```python
from build123d import *

# Parameters (mm, degrees)
SKETCH1_W                = 13
SKETCH1_H                = 6.8
BOSS_EXTRUDE1_DEPTH      = 6.4
SKETCH2_W                = 3.286897276
SKETCH2_H                = 0.917770019
SKETCH2_W_2              = 3.564362631
BOSS_EXTRUDE2_DEPTH      = 0.1
BOSS_EXTRUDE2_DEPTH_BACK = 6.9
SKETCH3_W                = 13
SKETCH3_H                = 7
SKETCH3_W_2              = 6.2
SKETCH3_H_2              = 3.9
BOSS_EXTRUDE3_DEPTH      = 0.1
SKETCH4_W                = 3.95
SKETCH4_H                = 3.9
BOSS_EXTRUDE4_DEPTH      = 4.87
SKETCH5_W                = 1.121207547
SKETCH5_H                = 2.774653545
SKETCH5_W_2              = 1.301952817
SKETCH5_H_2              = 2.838684011
SKETCH5_W_3              = 1.216578862
BOSS_EXTRUDE5_DEPTH      = 4


with BuildPart() as part:
    # Sketch1 → Boss-Extrude1 (new body)
    with BuildSketch(Plane(origin=(0, 0, 0), x_dir=(1, 0, 0), z_dir=(0, 1, 0))):
        with Locations((0.47556701, 2.025979381)):
            Rectangle(SKETCH1_W, SKETCH1_H)
    extrude(amount=BOSS_EXTRUDE1_DEPTH)

    # Sketch2 → Boss-Extrude2 (add, two sides)
    with BuildSketch(Plane.XY.offset(1.374020619)) as boss_extrude2_sk:
        Polygon((6.97556701, 6.4), (-6.02443299, 6.4), (-6.02443299, 1.631253573), (-0.351493181, 1.631253573), (-0.351493181, 3.2), (1.15322278, 3.2), (1.15322278, 1.631253573), (6.97556701, 1.631253573), align=None)
        with Locations((-3.350253358, 2.74111499)):
            Rectangle(SKETCH2_W, SKETCH2_H, mode=Mode.SUBTRACT)
        with Locations((4.087952491, 2.74111499)):
            Rectangle(SKETCH2_W_2, SKETCH2_H, mode=Mode.SUBTRACT)
    extrude(amount=BOSS_EXTRUDE2_DEPTH)
    extrude(boss_extrude2_sk.sketch, amount=-BOSS_EXTRUDE2_DEPTH_BACK)

    # Sketch3 → Boss-Extrude3 (add)
    with BuildSketch(Plane(origin=(0, 6.4, 0), x_dir=(1, 0, 0), z_dir=(0, 1, 0))):
        with Locations((0.47556701, 2.025979381)):
            Rectangle(SKETCH3_W, SKETCH3_H)
        with Locations((0.47556701, 2.025979381)):
            Rectangle(SKETCH3_W_2, SKETCH3_H_2, mode=Mode.SUBTRACT)
    extrude(amount=BOSS_EXTRUDE3_DEPTH)

    # Sketch4 → Boss-Extrude4 (add)
    with BuildSketch(Plane(origin=(0, 6.4, 0), x_dir=(1, 0, 0), z_dir=(0, 1, 0))):
        with Locations((-0.64943299, 2.025979381)):
            Rectangle(SKETCH4_W, SKETCH4_H)
    extrude(amount=BOSS_EXTRUDE4_DEPTH)

    # Sketch5 → Boss-Extrude5 (add)
    with BuildSketch(Plane.XZ):
        with Locations((0.400527608, -1.983292404)):
            Rectangle(SKETCH5_W, SKETCH5_H)
        with Locations((-4.182649421, -2.004635893)):
            Rectangle(SKETCH5_W_2, SKETCH5_H_2)
        with Locations((5.059081231, -2.036651126)):
            Rectangle(SKETCH5_W_3, SKETCH5_H)
    extrude(amount=BOSS_EXTRUDE5_DEPTH)


solid = part.part
```
Build history of the part. All positions in model axes, mm. A direction names the side the tool comes from. Coordinates: 2 decimals unless noted, no trailing zeros. Order: outer loops, then holes, each group sorted by start corner. A loop starts at its lowest first (then second) coordinate and runs counter-clockwise, first axis right, second up. Notation, with made-up numbers: (85, 83.25) -> (112, 83.25) arc R16 ccw to (112, 96.25) -> close; hole circle Ø10 at (-16.75, -33). An arc over 180 degrees is marked (long way). Answer in a Markdown table with one row per item. Add a question column.
Q1. Band-saw the part on C-C, the plane x = -3. List the corners of the cut face in (y, z), then the cut area to 3 significant figures.
Q2. Which spindle directions (+Z, -Z, +X, -X, +Y, -Y) get a long thin tool onto all of the face, cutting with end or side? Do faces 1 (the face through (4, 3, 1.374)), 2 (the face through (4.451, -2, -2)), 3 (the face through (5, -2, -3.424)). Say none if no direction does.
Q3. Band-saw the part on A-A, the plane y = -2.5. List the corners of the cut face in (x, z).
Q4. Band-saw the part on B-B, the plane z = -2.5. List the corners of the cut face in (x, y).
Q5. Wall check: line 1 along X through (y, z) = (-1.75, -1.5); line 2 along Z through (x, y) = (0.5, -2.5); line 3 along Y through (x, z) = (0, -4.5). Give the ranges that are in metal, low to high. Write a range as [from, to].
Q6. Band-saw the part on D-D, the plane y = 2.5. List the corners of the cut face in (x, z).
Q7. Drop flat-ended pins along their axis: pin 1 (2 mm diameter, centred on y = -3, z = -2.5, fed in from -X); pin 2 (2 mm diameter, centred on x = 2.5, z = -3.5, fed in from +Y); pin 3 (1 mm diameter, centred on x = 5.5, y = -1.5, fed in from +Z). Give the stop position or say it passes through.
Q8. Mould opens along Z. For faces 4 (the face through (-1, 9, -0.076)), 5 (the face through (2, 6.4, -2)), 6 (the face through (-3, 3, -5.426)) say: +Z half, -Z half, draft (parallel to the pull), parting line (faces both ways), or undercut.
Answers follow:
| question | item | result |
|---|---|---|
| 1 | outline | (0, -5.43) -> (1.63, -5.43) -> (1.63, -5.53) -> (2.28, -5.53) -> (2.28, -5.43) -> (3.2, -5.43) -> (3.2, -5.53) -> (6.5, -5.53) -> (6.5, 1.47) -> (3.2, 1.47) -> (3.2, 1.37) -> (2.28, 1.37) -> (2.28, 1.47) -> (1.63, 1.47) -> (1.63, 1.37) -> (0, 1.37) -> close |
| 1 | area | 45.0 mm^2 |
| 2 | face 1 | +Z |
| 2 | face 2 | +Z, -Z, -Y |
| 2 | face 3 | -Z, +X, -X, -Y |
| 3 | outline | (-4.83, -3.42) -> (-3.53, -3.42) -> (-3.53, -0.59) -> (-4.83, -0.59) -> close; (-0.16, -3.37) -> (0.96, -3.37) -> (0.96, -0.6) -> (-0.16, -0.6) -> close; (4.45, -3.42) -> (5.67, -3.42) -> (5.67, -0.65) -> (4.45, -0.65) -> close |
| 4 | outline | (-6.02, 0) -> (-4.83, 0) -> (-4.83, -4) -> (-3.53, -4) -> (-3.53, 0) -> (-0.16, 0) -> (-0.16, -4) -> (0.96, -4) -> (0.96, 0) -> (4.45, 0) -> (4.45, -4) -> (5.67, -4) -> (5.67, 0) -> (6.98, 0) -> (6.98, 6.5) -> (3.58, 6.5) -> (3.58, 6.4) -> (1.33, 6.4) -> (1.33, 11.27) -> (-2.62, 11.27) -> (-2.62, 6.5) -> (-6.02, 6.5) -> close |
| 5 | line 1 | [-4.83, -3.53], [-0.16, 0.96], [4.45, 5.67] |
| 5 | line 2 | [-3.37, -0.6] |
| 5 | line 3 | [0, 6.5] |
| 6 | outline | (-6.02, -5.53) -> (-4.99, -5.53) -> (-4.99, -5.43) -> (-1.71, -5.43) -> (-1.71, -5.53) -> (-0.35, -5.53) -> (-0.35, -5.43) -> (1.15, -5.43) -> (1.15, -5.53) -> (2.31, -5.53) -> (2.31, -5.43) -> (5.87, -5.43) -> (5.87, -5.53) -> (6.98, -5.53) -> (6.98, 1.47) -> (5.87, 1.47) -> (5.87, 1.37) -> (2.31, 1.37) -> (2.31, 1.47) -> (1.15, 1.47) -> (1.15, 1.37) -> (-0.35, 1.37) -> (-0.35, 1.47) -> (-1.71, 1.47) -> (-1.71, 1.37) -> (-4.99, 1.37) -> (-4.99, 1.47) -> (-6.02, 1.47) -> close |
| 7 | pin 1 | x = -4.83 |
| 7 | pin 2 | y = 6.5 |
| 7 | pin 3 | z = -0.65 |
| 8 | face 4 | +Z half |
| 8 | face 5 | undercut |
| 8 | face 6 | -Z half |
